Here's how the part is built. I have some questions about the finished solid (model axes, mm). A direction names the side the tool comes from. Coordinates: 2 decimals unless noted, no trailing zeros. Write each loop counter-clockwise with the first axis right and the second up, starting at its lowest first coordinate (ties: lowest second). Pieces come first, ordered by that corner, then holes.
(1) Please list where these lines run through material, in increasing order: probe 1 along Y at (x, z) = (18, 0.4); probe 2 along Y at (x, z) = (18, -0.7); probe 3 along Y at (x, z) = (15.75, 2.75).
(2) Imagine slicing it at A-A, the plane x = 18. List the corners of the cut face in (y, z) for me.
(3) Thinking about a two-plate mould opening in Y: for faces 4 (the flat face through (16, 80, 1)), 5 (the flat face through (15, 5, 1)), 6 (the flat face through (16, 65, 6)), which applies, released by +Y, released by -Y, zero draft, split by the parting line, or undercut?
(4) Imagine slicing it at C-C, the plane x = 10. List the corners of the cut face in (y, z) for me.
(5) Which directions (+Z, -Z, +X, -X, +Y, -Y) give clear straight access to the entire face, cutting with the end or side of a thin tool? Please do faces 1 (the flat face through (18, 5, 0)), 2 (the flat face through (15, -6, 1)), 3 (the flat face through (18, 6, 1)).
(6) Imagine slicing it at B-B, the plane y = 17.5. List the corners of the cut face in (x, z) for me, plus the area to 3 significant figures.
(7) Imagine slicing it at D-D, the plane x = 1. List the corners of the cut face in (y, z) for me, plus the area to 3 significant figures.
(8) For pin 1 Ø1.5 at (x, z) = (14, 2) entering from -Y; pin 2 Ø2 at (y, z) = (-6, 1) entering from -X; pin 3 Ø1 at (y, z) = (34, 1) entering from +X; pin 4 Ø1.5 at (x, z) = (8, 3) entering from -Y, each with a flat end and sliding along its axis, tell me the tip position at first contact or that it passes through.
```python
from build123d import *

# Parameters (mm, degrees)
SKETCH_1_R             = 1.85
EXTRUDE_1_DEPTH        = 2
CUT_EXTRUDE_START      = -4
SKETCH_4_W             = 6
SKETCH_4_H             = 3
SKETCH_4_H_2           = 7
CUT_EXTRUDE_2_DEPTH    = 2
EXTRUDE_2_DEPTH        = 2
SKETCH_5_W             = 10
SKETCH_5_H             = 30
EXTRUDE_3_DEPTH        = 2
CUT_EXTRUDE_3_DEPTH    = 10
PATTERN_LINEAR_1_COUNT = 21
PATTERN_LINEAR_1_PITCH = 1.414


with BuildPart() as part:
    # 草图1 → 凸台-拉伸1 (new, symmetric)
    with BuildSketch(Plane.XY):
        with BuildLine():
            Line((20, 6), (16, 6))
            Line((16, 6), (15, 6))
            Line((15, 6), (15, 3))
            Line((15, 3), (3, 3))
            Line((3, 3), (-3, 3))
            Line((-3, 3), (-3, 0))
            ThreePointArc((-3, 0), (-2.121320344, -2.121320344), (0, -3))
            Line((0, -3), (15, -3))
            Line((15, -3), (15, -10))
            Line((15, -10), (16, -10))
            Line((16, -10), (20, -10))
            Line((20, -10), (20.5, -10))
            Line((20.5, -10), (21, -10))
            Line((21, -10), (21, -3))
            Line((21, -3), (21, 3))
            Line((21, 3), (21, 6))
            Line((21, 6), (20, 6))
        make_face()
        with Locations((18, 0)):
            Circle(SKETCH_1_R, mode=Mode.SUBTRACT)
    extrude(amount=EXTRUDE_1_DEPTH, both=True)

    # 草图4 → 切除-拉伸2 (cut)
    with BuildSketch(Plane.XY.offset(2).offset(CUT_EXTRUDE_START)):
        with Locations((18, 4.5)):
            Rectangle(SKETCH_4_W, SKETCH_4_H)
        with Locations((18, -6.5)):
            Rectangle(SKETCH_4_W, SKETCH_4_H_2)
    extrude(amount=CUT_EXTRUDE_2_DEPTH, mode=Mode.SUBTRACT)

    # 草图1<3> → 凸台-拉伸2 (add)
    with BuildSketch(Plane.XY):
        with BuildLine():
            Line((-3, 3), (3, 3))
            Line((3, 3), (3, 48.757359313))
            Line((3, 48.757359313), (15.121320344, 60.878679656))
            Line((15.121320344, 60.878679656), (15.121320344, 69.363961031))
            Line((15.121320344, 69.363961031), (10.878679656, 65.121320344))
            Line((10.878679656, 65.121320344), (-2.121320344, 52.121320344))
            ThreePointArc((-2.121320344, 52.121320344), (-2.771638598, 51.148050297), (-3, 50))
            Line((-3, 50), (-3, 3))
        make_face()
    extrude(amount=EXTRUDE_2_DEPTH)

    # 草图5 → 凸台-拉伸3 (add)
    with BuildSketch(Plane(origin=(15.121320344, 0, 0), x_dir=(0, 0, -1), z_dir=(1, 0, 0))):
        with Locations((-1, 65)):
            Rectangle(SKETCH_5_W, SKETCH_5_H)
    extrude(amount=EXTRUDE_3_DEPTH)

    # 草图6 → 切除-拉伸3 (cut)
    with BuildSketch(Plane.XY.offset(6)):
        Polygon((17.121320344, 80), (16.414213562, 79.292893219), (17.121320344, 78.585786438), align=None)
    cut_extrude_3 = extrude(amount=-CUT_EXTRUDE_3_DEPTH, mode=Mode.SUBTRACT)

    # 阵列(线性)1: 切除-拉伸3 ×21
    with Locations(*[(0, -i * PATTERN_LINEAR_1_PITCH, 0) for i in range(1, PATTERN_LINEAR_1_COUNT)]):
        add(cut_extrude_3, mode=Mode.SUBTRACT)


solid = part.part
```
Recorded:
1. probe 1: y = -10 to -1.85, 1.85 to 6
1. probe 2: y = -3 to -1.85, 1.85 to 3
1. probe 3: y = 50 to 80
2. outline: (-10, 0) - (-3, 0) - (-3, -2) - (-1.85, -2) - (-1.85, 2) - (-10, 2) - close; (1.85, -2) - (3, -2) - (3, 0) - (6, 0) - (6, 2) - (1.85, 2) - close
3. face 4: released by +Y
3. face 5: undercut
3. face 6: zero draft
4. outline: (-3, -2) - (3, -2) - (3, 2) - (-3, 2) - close; (55.76, 0) - (64.24, 0) - (64.24, 2) - (55.76, 2) - close
5. face 1: -Z, +X, -X
5. face 2: +Z, -Z, -X, -Y
5. face 3: +Z, -Z, +X
6. outline: (-3, 0) - (3, 0) - (3, 2) - (-3, 2) - close
6. area: 12.0 mm2
7. outline: (-3, -2) - (3, -2) - (3, 0) - (55.24, 0) - (55.24, 2) - (-3, 2) - close
7. area: 128 mm2
8. pin 1: stops at y = -3
8. pin 2: stops at x = 15
8. pin 3: stops at x = 3
8. pin 4: passes through
